```python
from build123d import *

# Parameters (mm, degrees)
SKETCH1_W           = 75
SKETCH1_H           = 4
BOSS_EXTRUDE1_DEPTH = 2.5
SKETCH2_R           = 1.15
CUT_EXTRUDE1_DEPTH  = 3
SKETCH3_W           = 30
SKETCH3_H           = 4
BOSS_EXTRUDE2_DEPTH = 0.6
SKETCH2_2_R         = 1.15
CUT_EXTRUDE2_DEPTH  = 76.148186938
SKETCH4_R           = 1.15
CUT_EXTRUDE3_DEPTH  = 76.170539442


with BuildPart() as part:
    # Sketch1 → Boss-Extrude1 (new body)
    with BuildSketch(Plane.XY):
        with Locations((37.5, 2)):
            Rectangle(SKETCH1_W, SKETCH1_H)
    extrude(amount=BOSS_EXTRUDE1_DEPTH)

    # Sketch2 → Cut-Extrude1 (cut)
    with BuildSketch(Plane(origin=(0, 0, 0), x_dir=(-1, 0, 0), z_dir=(0, 0, -1))):
        with Locations((-37.5, 2)):
            Circle(SKETCH2_R)
    extrude(amount=-CUT_EXTRUDE1_DEPTH, mode=Mode.SUBTRACT)

    # Sketch3 → Boss-Extrude2 (add)
    with BuildSketch(Plane(origin=(0, 0, 0), x_dir=(-1, 0, 0), z_dir=(0, 0, -1))):
        with Locations((-37.5, 2)):
            Rectangle(SKETCH3_W, SKETCH3_H)
    extrude(amount=BOSS_EXTRUDE2_DEPTH)

    # Sketch2<2> → Cut-Extrude2 (cut, through all)
    with BuildSketch(Plane(origin=(0, 0, 0), x_dir=(-1, 0, 0), z_dir=(0, 0, -1))):
        with Locations((-37.5, 2)):
            Circle(SKETCH2_2_R)
    extrude(amount=CUT_EXTRUDE2_DEPTH, mode=Mode.SUBTRACT)

    # Sketch4 → Cut-Extrude3 (cut, through all)
    with BuildSketch(Plane.XY.offset(2.5)):
        with Locations((24.5, 2.076531631)):
            Circle(SKETCH4_R)
        with Locations((50.5, 2.076531631)):
            Circle(SKETCH4_R)
    extrude(amount=-CUT_EXTRUDE3_DEPTH, mode=Mode.SUBTRACT)


solid = part.part
```
Here's how the part is built. I have some questions about the finished solid (model axes, mm). A direction names the side the tool comes from. Give positions to 0.01 mm unless a question says otherwise; leave off trailing zeros. Write each loop counter-clockwise with the first axis right and the second up, starting at its lowest first coordinate (ties: lowest second). Pieces come first, ordered by that corner, then holes. Notation, with made-up numbers: M -38.5,22.25 L 4.5,22.25 A13 ccw 4.5,42.25 Z; hole C -10.5,63.25 d4. An arc over 180 degrees is marked long. Put each result on its own line as item: value. Start each with the question number.
Item 1: Thinking about a two-plate mould opening in Y: for faces 4 (the cylindrical face through (23.7, 2.9, 1)), 5 (the flat face through (38, 0, 1)), 6 (the flat face through (37.7, 0.7, -0.6)), which applies, +Y half, -Y half, draft (parallel to the pull), parting line (faces both ways), or undercut?
Item 2: If we section it at B-B, the plane z = 1.85: Write out the boundary of the cut face in (x, y).
Item 3: On a 3-axis mill with a long thin cutter (end or side, diameter ignored), from which of +Z, -Z, +X, -X, +Y, -Y can I reach the whole of each face in a straight line? I mean faces 1 (the flat face through (64, 2, 0)), 2 (the flat face through (11, 2, 0)), 3 (the flat face through (75, 2, 1)). Say none if no direction works.
Item 4: Will this pin go through, and if not, where does the flat tip stop? pin 1 (1.2 mm diameter, centred on x = 12, y = 3, fed in from -Z).
Item 5: If we section it at C-C, the plane x = 37: Write out the boundary of the cut face in (y, z).
Item 6: I need wall thicknesses on L1, parallel to X at y = 2, z = -0.1; L2, parallel to X at y = 2.15, z = 2.05; L3, parallel to Y at x = 24.5, z = 0.7. Which ranges of each line are inside material? Lowest first, please. Write a range as from..to.
Item 7: If we section it at A-A, the plane x = 24.5: Write out the boundary of the cut face in (y, z), then the cut area to 3 significant figures.
Values:
1. face 4: undercut
1. face 5: -Y half
1. face 6: draft
2. outline: M 0,0 L 75,0 L 75,4 L 0,4 Z; hole C 24.5,2.08 d2.3; hole C 37.5,2 d2.3; hole C 50.5,2.08 d2.3
3. face 1: -Z, +X, +Y, -Y
3. face 2: -Z, -X, +Y, -Y
3. face 3: +Z, -Z, +X, +Y, -Y
4. pin 1: z = 0
5. outline: M 0,-0.6 L 0.96,-0.6 L 0.96,2.5 L 0,2.5 Z; M 3.04,-0.6 L 4,-0.6 L 4,2.5 L 3.04,2.5 Z
6. L1: 22.5..23.35, 25.65..36.35, 38.65..49.35, 51.65..52.5
6. L2: 0..23.35, 25.65..36.36, 38.64..49.35, 51.65..75
6. L3: 0..0.93, 3.23..4
7. outline: M 0,-0.6 L 0.93,-0.6 L 0.93,2.5 L 0,2.5 Z; M 3.23,-0.6 L 4,-0.6 L 4,2.5 L 3.23,2.5 Z
7. area: 5.27 mm²
